CAD build for the part. Positions are in the model's coordinates, mm. Face numbers are marked on the shaded views. Coordinates: 2 decimals unless noted, no trailing zeros. Write each loop counter-clockwise with the first axis right and the second up, starting at its lowest first coordinate (ties: lowest second). Pieces come first, ordered by that corner, then holes.
```python
from build123d import *

# Parameters (mm, degrees)
SKETCH1_R           = 7.5
SKETCH1_R_2         = 6.75
BOSS_EXTRUDE1_DEPTH = 70
FILLET2_R           = 0.37
SKETCH8_R           = 9.678517052
BOSS_EXTRUDE6_DEPTH = 2
SKETCH9_R           = 6.75
CUT_EXTRUDE2_DEPTH  = 72
SKETCH10_R          = 2
CUT_EXTRUDE3_DEPTH  = 10


with BuildPart() as part:
    # Sketch1 → Boss-Extrude1 (new body)
    with BuildSketch(Plane.XY):
        Circle(SKETCH1_R)
        Circle(SKETCH1_R_2, mode=Mode.SUBTRACT)
    extrude(amount=BOSS_EXTRUDE1_DEPTH)

    # Fillet2
    fillet2_edges = [part.edges().sort_by_distance(p)[0] for p in [
        (-7.5, 0, 0),
        (-6.75, 0, 0),
    ]]
    fillet(fillet2_edges, radius=FILLET2_R)

    # Sketch8 → Boss-Extrude6 (add)
    with BuildSketch(Plane(origin=(-15.511368661, 0, 33.264237441), x_dir=(0, -1, 0), z_dir=(-0.4226182617407003, 0, 0.9063077870366496))):
        with Locations(Location((0, 16.981195542, 0), (0, 0, 90))):
            Circle(SKETCH8_R)
    extrude(amount=BOSS_EXTRUDE6_DEPTH)

    # Sketch9 → Cut-Extrude2 (cut)
    with BuildSketch(Plane.XY):
        Circle(SKETCH9_R)
    extrude(amount=CUT_EXTRUDE2_DEPTH, mode=Mode.SUBTRACT)

    # Sketch10 → Cut-Extrude3 (cut)
    with BuildSketch(Plane(origin=(0, 0, 0), x_dir=(0, 0, -1), z_dir=(1, 0, 0))):
        with Locations(Location((-21.875209452, 0, 0), (0, 0, 180))):
            Circle(SKETCH10_R)
    extrude(amount=CUT_EXTRUDE3_DEPTH, mode=Mode.SUBTRACT)


solid = part.part
```
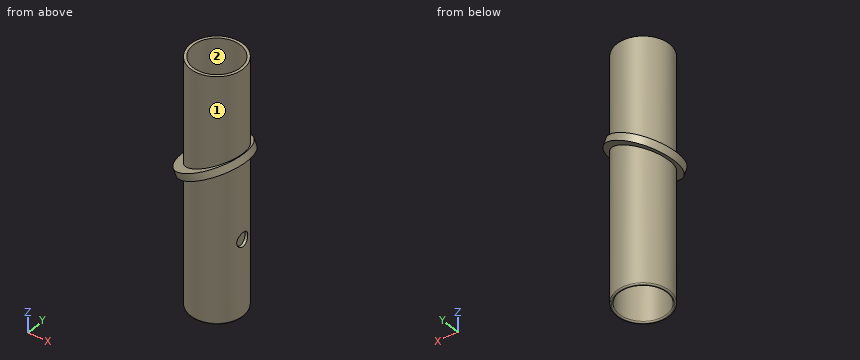
Item 1: Flat gauge pins, fed straight in: pin 1 Ø8 at (y, z) = (7.5, 20) entering from +X; pin 2 Ø4.5 at (y, z) = (0, 21.88) entering from +X; pin 3 Ø3 at (x, z) = (1, 59) entering from +Y; pin 4 Ø2 at (x, y) = (3, 4) entering from +Z. Where does each tip first touch, or does it go through?
Item 2: Saw through at A-A, the plane y = 0. State how many separate pieces and enclosed holes the cut face has, and give its area (3 significant figures).
Item 3: Two-plate mould, pull along Y, no slides. Class the marked faces 1 and 2: +Y half, -Y half, draft (parallel to the pull), parting line (faces both ways), or undercut.
Item 4: Wall check: line 1 along Y through (x, z) = (0, 57.5); line 2 along Y through (x, z) = (-2.75, 20); line 3 along X through (y, z) = (3, 29.5). Give the ranges that are in metal, low to high.
Item 5: Saw through at C-C, the plane z = 23. Write the cut outline in (x, y).
Item 6: Saw through at B-B, the plane z = 34. Write the cut outline in (x, y), and give its area (3 significant figures).
Working result:
1. pin 1: stops at x = 6.63
1. pin 2: stops at x = 7.5
1. pin 3: stops at y = 7.5
1. pin 4: passes through
2. separate pieces: 3
2. enclosed holes: 0
2. area: 107 mm2
3. face 1: parting line
3. face 2: undercut
4. line 1: y = -7.5 to -6.75, 6.75 to 7.5
4. line 2: y = -6.98 to -6.16, 6.16 to 6.98
4. line 3: x = -6.87 to -6.05, 6.05 to 6.87
5. outline: (6.54, -1.65) arc R6.75 cw (long way) to (6.54, 1.65) - (7.32, 1.65) arc R7.5 ccw (long way) to (7.32, -1.65) - close
6. outline: circle Ø15 at (0, 0); hole circle Ø13.5 at (0, 0)
6. area: 33.6 mm2
